Geometry: final body of the model. Coordinates: model frame, mm. Face numbers are marked on the shaded views. A direction names the side the tool comes from. Coordinates: 2 decimals unless noted, no trailing zeros. Order: outer loops, then holes, each group sorted by start corner. A loop starts at its lowest first (then second) coordinate and runs counter-clockwise, first axis right, second up. Notation, with made-up numbers: (84, 56.5) -> (127, 56.5) arc R8 ccw to (127, 70.5) -> close; hole circle Ø5 at (4, 71.25). An arc over 180 degrees is marked (long way). Answer in a Markdown table with one row per item. Add a question column.
1) Set-up query: the marked faces 5, 6 and 7. Return all of +Z, -Z, +X, -X, +Y, -Y with unobstructed straight access to the full face (end or side cutting, diameter ignored); none if empty.
2) Ray query, line 1 (Z direction, x = 1.95, y = 0); line 2 (Y direction, x = 1.9, z = 0); line 3 (Y direction, x = 0.1, z = 7.25). Return the intervals inside material, ascending. Write a range as from..to.
3) Contact query for a flat-ended pin moving along its axis: P1, Ø1.5, axis at x = 0.5, y = 5.5, coming from the +Z side. Output: stop coordinate, or through.
4) Section query C-C on y = 4. Return the cut outline in (x, z), then the cut area to 3 significant figures.
5) Section query A-A on y = 0. Return the cut outline in (x, z).
6) Pull-direction query (Z, two-part tool) for the marked faces 1, 2, 3 and 4; classes: +Z half, -Z half, draft (parallel to the pull), parting line (faces both ways), or undercut.
7) Section query B-B on z = -1.5. Return the cut outline in (x, y).
```python
from build123d import *

# Parameters (mm, degrees)
BASPROSKE_W         = 2.5
BASPROSKE_H         = 8
TOOTHCUT_DEPTH      = 12.586630226
TEETHCUTS_COUNT     = 30
TEETHCUTS_ANGLE     = 348
BORSKE_R            = 3
BORE_DEPTH          = 50.0000508
EXTRUDE_1_DEPTH     = 2.5
SKETCH_2_R          = 0.5
CUT_EXTRUDE_1_DEPTH = 12.568528524


with BuildPart() as part:
    # BasProSke → Base-Revolve (revolve)
    with BuildSketch(Plane(origin=(0, 0, 0), x_dir=(1, 0, 0), z_dir=(0, 1, 0)), mode=Mode.PRIVATE) as base_revolve_sk:
        with Locations((1.25, 4)):
            Rectangle(BASPROSKE_W, BASPROSKE_H)
    revolve(base_revolve_sk.sketch.rotate(Axis((-10, 0, 0), (1, 0, 0)), 180), axis=Axis((-10, 0, 0), (1, 0, 0)))

    # TooCutSke → ToothCut (cut, through all)
    with BuildSketch(Plane(origin=(0, 0, 0), x_dir=(0, 0, -1), z_dir=(1, 0, 0))):
        with BuildLine():
            ThreePointArc((0.279013782, 6.868335119), (0, 6.874), (-0.279013782, 6.868335119))
            ThreePointArc((-0.279013782, 6.868335119), (-0.413500328, 7.452412324), (-0.661410108, 7.998098638))
            ThreePointArc((-0.661410108, 7.998098638), (0, 8.0254), (0.661410108, 7.998098638))
            ThreePointArc((0.661410108, 7.998098638), (0.413500328, 7.452412324), (0.279013782, 6.868335119))
        make_face()
    toothcut = extrude(amount=TOOTHCUT_DEPTH, mode=Mode.SUBTRACT)

    # TeethCuts: ToothCut ×30 about axis
    teethcuts_axis = Axis((-10, 0, 0), (1, 0, 0))
    for i in range(1, TEETHCUTS_COUNT):
        add(toothcut.rotate(teethcuts_axis, i * TEETHCUTS_ANGLE / (TEETHCUTS_COUNT - 1)), mode=Mode.SUBTRACT)

    # BorSke → Bore (cut, symmetric)
    with BuildSketch(Plane(origin=(0, 0, 0), x_dir=(0, 0, -1), z_dir=(1, 0, 0))):
        with Locations(Location((0, 0, 0), (0, 0, 180))):
            Circle(BORSKE_R)
    extrude(amount=BORE_DEPTH, both=True, mode=Mode.SUBTRACT)

    # 草图1 → 凸台-拉伸1 (add, through all)
    with BuildSketch(Plane(origin=(2.5, 0, 0), x_dir=(0, 0, -1), z_dir=(1, 0, 0))):
        with BuildLine():
            Line((-2.236067977, 2), (2.236067977, 2))
            ThreePointArc((2.236067977, 2), (0, 3), (-2.236067977, 2))
        make_face()
    extrude(amount=-EXTRUDE_1_DEPTH)

    # 草图2 → 切除-拉伸1 (cut, through all)
    with BuildSketch(Plane(origin=(2.5, 0, 0), x_dir=(0, 0, -1), z_dir=(1, 0, 0))):
        with Locations((2.236067977, 2)):
            Circle(SKETCH_2_R)
        with Locations((-2.236067977, 2)):
            Circle(SKETCH_2_R)
    extrude(amount=-CUT_EXTRUDE_1_DEPTH, mode=Mode.SUBTRACT)


solid = part.part
```
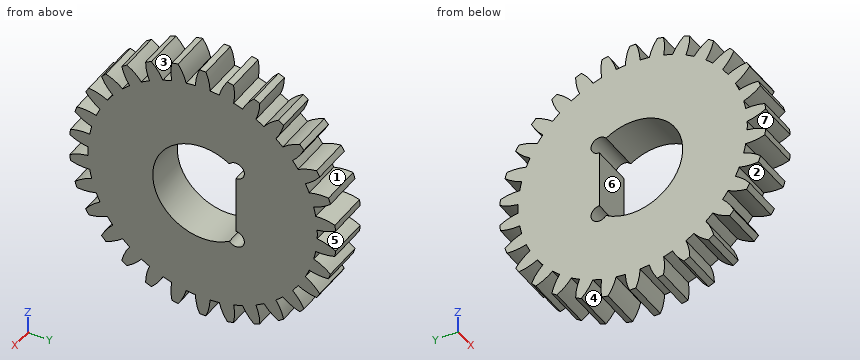
Result:
| question | item | result |
|---|---|---|
| 1 | face 5 | +X, -X, +Y |
| 1 | face 6 | +X, -X |
| 1 | face 7 | +X, -X, -Y |
| 2 | line 1 | -8..-3, 3..8 |
| 2 | line 2 | -6.87..-3, 2..6.87 |
| 2 | line 3 | -3.38..-2.94, -1.91..-1.14, -0.41..0.41, 1.14..1.91, 2.94..3.38 |
| 3 | P1 | z = 6.44 |
| 4 | outline | (0, -6.17) -> (2.5, -6.17) -> (2.5, 6.17) -> (0, 6.17) -> close |
| 4 | area | 30.9 mm2 |
| 5 | outline | (0, -8) -> (2.5, -8) -> (2.5, -3) -> (0, -3) -> close; (0, 3) -> (2.5, 3) -> (2.5, 8) -> (0, 8) -> close |
| 6 | face 1 | undercut |
| 6 | face 2 | undercut |
| 6 | face 3 | +Z half |
| 6 | face 4 | -Z half |
| 7 | outline | (0, -6.71) -> (2.5, -6.71) -> (2.5, -2.6) -> (0, -2.6) -> close; (0, 2) -> (2.5, 2) -> (2.5, 6.71) -> (0, 6.71) -> close |
